from build123d import *


with BuildPart() as part:
    # Sketch1 → Revolve1 (revolve)
    with BuildSketch(Plane.XY, mode=Mode.PRIVATE) as revolve1_sk:
        with BuildLine():
            Line((0.3, 5), (4.7, 5))
            ThreePointArc((4.7, 5), (4.912132034, 4.912132034), (5, 4.7))
            Line((5, 4.7), (5, 2.723209195))
            ThreePointArc((5, 2.723209195), (5.059312122, 2.544130036), (5.213795634, 2.43586131))
            Line((5.213795634, 2.43586131), (9.786204366, 1.06413869))
            ThreePointArc((9.786204366, 1.06413869), (9.940687878, 0.955869964), (10, 0.776790805))
            Line((10, 0.776790805), (10, 0))
            Line((10, 0), (4, 0.5))
            Line((4, 0.5), (0, 0.5))
            Line((0, 0.5), (0, 4.7))
            ThreePointArc((0, 4.7), (0.087867966, 4.912132034), (0.3, 5))
        make_face()
    revolve(revolve1_sk.sketch.rotate(Axis((10, -22.5, 0), (-1, 0, 0)), 90), axis=Axis((10, -22.5, 0), (-1, 0, 0)))


solid = part.part
Check sheet for the modelled part. Datum: model origin and axes. Units: mm. A direction names the side the tool comes from. Give positions to 0.01 mm unless a question says otherwise; leave off trailing zeros. Write each loop counter-clockwise with the first axis right and the second up, starting at its lowest first coordinate (ties: lowest second). Pieces come first, ordered by that corner, then holes. Notation, with made-up numbers: (-24, 8) -> (-16, 8) arc R21 cw to (-16, 44) -> close; hole circle Ø7 at (84.25, 40.25). An arc over 180 degrees is marked (long way). Write item = value, one per line.
Item 1: Gauge pin test, flat end, axial feed: pin 1 (4 mm diameter, centred on x = 8, z = 17.5, fed in from +Y). Record the tip position at first contact, or that the pin passes through.
Output:
pin_1 = -3.87
Item 2: Sectioned sample at A-A on z = 0. Record the boundary of the cut face in (x, y).
Output:
outline = (0, -49.7) arc R0.3 ccw to (0.3, -50) -> (4.7, -50) arc R0.3 ccw to (5, -49.7) -> (5, -47.72) arc R0.3 cw to (5.21, -47.44) -> (9.79, -46.06) arc R0.3 ccw to (10, -45.78) -> (10, -45) -> (4, -45.5) -> (0, -45.5) -> close; (0, 0.5) -> (4, 0.5) -> (10, 0) -> (10, 0.78) arc R0.3 ccw to (9.79, 1.06) -> (5.21, 2.44) arc R0.3 cw to (5, 2.72) -> (5, 4.7) arc R0.3 ccw to (4.7, 5) -> (0.3, 5) arc R0.3 ccw to (0, 4.7) -> close
Item 3: Sectioned sample at B-B on y = -22.5. Record the boundary of the cut face in (x, z), and give its area (3 significant figures).
Output:
outline = (0, -27.2) arc R0.3 ccw to (0.3, -27.5) -> (4.7, -27.5) arc R0.3 ccw to (5, -27.2) -> (5, -25.22) arc R0.3 cw to (5.21, -24.94) -> (9.79, -23.56) arc R0.3 ccw to (10, -23.28) -> (10, -22.5) -> (4, -23) -> (0, -23) -> close; (0, 23) -> (4, 23) -> (10, 22.5) -> (10, 23.28) arc R0.3 ccw to (9.79, 23.56) -> (5.21, 24.94) arc R0.3 cw to (5, 25.22) -> (5, 27.2) arc R0.3 ccw to (4.7, 27.5) -> (0.3, 27.5) arc R0.3 ccw to (0, 27.2) -> close
area = 60.4 mm^2
Item 4: Sectioned sample at D-D on x = 9. Record the boundary of the cut face in (y, z).
Output:
outline = circle Ø47.6 at (-22.5, 0); hole circle Ø45.17 at (-22.5, 0)
Item 5: Sectioned sample at C-C on x = 2.75. Record the boundary of the cut face in (y, z), and give its area (3 significant figures).
Output:
outline = circle Ø55 at (-22.5, 0); hole circle Ø46 at (-22.5, 0)
area = 714 mm^2
Item 6: Scan lines: probe 1 along Y at (x, z) = (0.85, 0); probe 2 along Z at (x, y) = (8.25, -17); probe 3 along Z at (x, y) = (1, -43.5). Record each from-to range of solid material in increasing order. Write a range as from..to.
Output:
probe_1 = -50..-45.5, 0.5..5
probe_2 = -23.39..-21.97, 21.97..23.39
probe_3 = -17.76..-9.38, 9.38..17.76
Item 7: Tool access check on faces 1 (the flat face through (5, 2, -8)), 2 (the cylindrical face through (1.972, -45.304, 2.994)), 3 (the cylindrical face through (2.53, -30.76, -26.23)). Record the directions out of +Z, -Z, +X, -X, +Y, -Y that give a thin tool (end or side, any length) a straight path to the whole face; none if there is none.
Output:
face_1 = +X
face_2 = -X
face_3 = +X, -X
Item 8: Release check for a two-part mould opening along Y. For faces 4 (the conical face through (8.96, -0.45, 4.9)), 5 (the conical face through (9.56, -29.6, -22.54)), 6 (the flat face through (0, -45, 6)) record: +Y half, -Y half, draft (parallel to the pull), parting line (faces both ways), or undercut.
Output:
face_4 = undercut
face_5 = parting line
face_6 = draft
